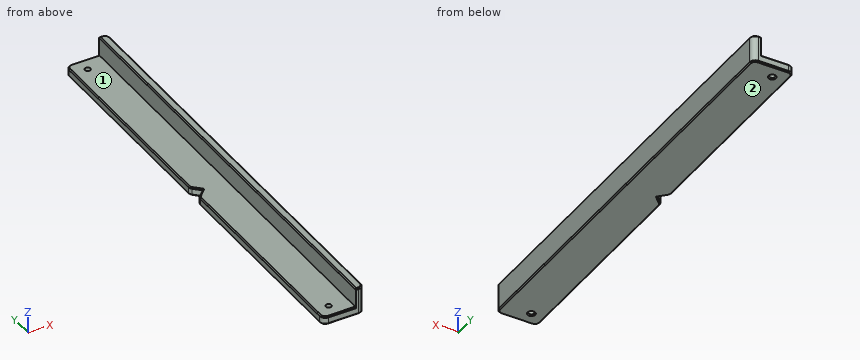
Autodesk Fusion 360 part; units mm, degrees
sketch "Sketch1" plane through (0, 0, 0) normal (0, 0, 1) x (1, 0, 0) in component "bed_hole_marking_template_x1_Rev2"
  line L0 (7.5, -80) -> (-7.5, -80)
  line L1 (-7.5, -80) -> (-7.5, 80)
  line L2 (-7.5, 80) -> (7.5, 80)
  line L3 (7.5, 80) -> (7.5, -80)
  line L4 (7.5, -80) -> (-7.5, 80) construction
  line L5 (-7.5, -80) -> (7.5, 80) construction
  line L6 (-4.5, -0.0061) -> (-7.5, 2.9939)
  line L7 (0, 0) -> (-10, 0) construction
  circle A0 centre (-2.5, 75) radius 1
  line L8 (-4.5, 0.0061) -> (-7.5, -2.9939)
  line L9 (4.5, 80) -> (4.5, -80)
  circle A1 centre (-2.5, -75) radius 1
  point P0 (-2.5, -75)
  dimension "d1" = 15
  dimension "d2" = 160
  dimension "d3" = 135
  dimension "d4" = 2
  dimension "d5" = 5
  dimension "d6" = 5
  dimension "d7" = 4.5
  dimension "d8" = 3
extrude "Extrude1" add sketch "Sketch1" against normal blind 3 contours L0 L2 L3 L9 | L0 L1 L2 L6 L8 L9 in component "bed_hole_marking_template_x1_Rev2"
extrude "Extrude2" add sketch "Sketch1" along normal blind 7 contours L0 L2 L3 L9 in component "bed_hole_marking_template_x1_Rev2"
fillet "Fillet1" radius 2 6 edges at (-7.5, 80, -1.5) (7.5, 80, 2) (-7.5, -80, -1.5) (7.5, -80, 2) (-7.5, 2.9939, -1.5) (-7.5, -2.9939, -1.5) in component "bed_hole_marking_template_x1_Rev2"
chamfer "Chamfer1" distance 0.4 angle 45 31 edges at (7.5, 0, 7) (6.9142, -79.4142, 7) (5, -80, 7) (5, 80, 7) (6.9142, 79.4142, 7) (4.5, 0, 7) (-0.5, -80, 0) (-6.9142, -79.4142, 0) (-7.5, -40.9112, 0) (-7.3478, -3.057, 0) (-5.7101, -1.2041, 0) (-7.5, 40.9112, 0) (-7.3478, 3.057, 0) (-5.7101, 1.2041, 0) (-0.5, 80, 0) (-6.9142, 79.4142, 0) (0, 80, -3) (-6.9142, 79.4142, -3) (-7.5, 40.9112, -3) (-7.3478, 3.057, -3) (-5.7101, 1.2041, -3) (-5.7101, -1.2041, -3) (-7.3478, -3.057, -3) (-7.5, -40.9112, -3) (-6.9142, -79.4142, -3) (0, -80, -3) (6.9142, -79.4142, -3) (7.5, 0, -3) (6.9142, 79.4142, -3) (-3.4323, 74.6384, -3) (-3.4323, -75.3616, -3) in component "bed_hole_marking_template_x1_Rev2"
component "bed_hole_marking_template_x1_Rev2" placed x (1, 0, 0) y (0, 1, 0) z (0, 0, 1) at (0, 0, 0)
The model under review builds one solid part; all positions refer to its coordinate system, in mm. Face numbers are marked on the shaded views. A direction names the side the tool comes from. Round coordinates to 2 decimals unless told otherwise and drop trailing zeros. Write each loop counter-clockwise with the first axis right and the second up, starting at its lowest first coordinate (ties: lowest second). Pieces come first, ordered by that corner, then holes. Notation, with made-up numbers: (49, -10) -> (58, -10) arc R12 cw to (58, 1) -> close; hole circle Ø10 at (-26, 7). An arc over 180 degrees is marked (long way). Answer as a JSON object with one key per item and string values.
1. To check wall thickness, follow line 1 along Y through (x, z) = (-2.5, -1.9); line 2 along X through (y, z) = (75, -1); line 3 along X through (y, z) = (28.5, 5.25). State the ranges of each line that lie inside material, in increasing order.
Results found:
{"line 1": "y = -80 to -76, -74 to 74, 76 to 80", "line 2": "x = -7.5 to -3.5, -1.5 to 7.5", "line 3": "x = 4.5 to 7.5"}
2. We need section B-B on z = 3.25. State the section outline as (x, y) points.
Results found:
{"outline": "(4.5, -80) -> (5.5, -80) arc R2 ccw to (7.5, -78) -> (7.5, 78) arc R2 ccw to (5.5, 80) -> (4.5, 80) -> close"}
3. We need section A-A on y = -7.5. State the section outline as (x, z) points.
Results found:
{"outline": "(-7.5, -2.6) -> (-7.1, -3) -> (7.1, -3) -> (7.5, -2.6) -> (7.5, 6.6) -> (7.1, 7) -> (4.9, 7) -> (4.5, 6.6) -> (4.5, 0) -> (-7.1, 0) -> (-7.5, -0.4) -> close"}
4. We need section C-C on x = 3. State the section outline as (y, z) points, and give its area (3 significant figures).
Results found:
{"outline": "(-80, -2.6) -> (-79.6, -3) -> (79.6, -3) -> (80, -2.6) -> (80, -0.4) -> (79.6, 0) -> (-79.6, 0) -> (-80, -0.4) -> close", "area": "480 mm^2"}
5. Machinability: for the marked faces 1 and 2, which of the approach directions +Z, -Z, +X, -X, +Y, -Y give a long, thin tool a straight path to every point of the face, cutting with its end or side? Answer none if there is none.
Results found:
{"face 1": "+Z, -X, +Y, -Y", "face 2": "-Z, +X, -X, +Y, -Y"}
6. Clearance check with flat-ended pins moving along their axes: pin 1 (1.5 mm diameter, centred on x = -3, z = 2, fed in from -Y); pin 2 (2.5 mm diameter, centred on x = -2.5, y = 75, fed in from +Z); pin 3 (2 mm diameter, centred on y = -17.5, z = 5, fed in from -X); pin 4 (3 mm diameter, centred on x = 4, y = 53.5, fed in from +Z). State where each tip first meets the part, or that it passes through.
Results found:
{"pin 1": "passes through", "pin 2": "stops at z = 0", "pin 3": "stops at x = 4.5", "pin 4": "stops at z = 7"}
